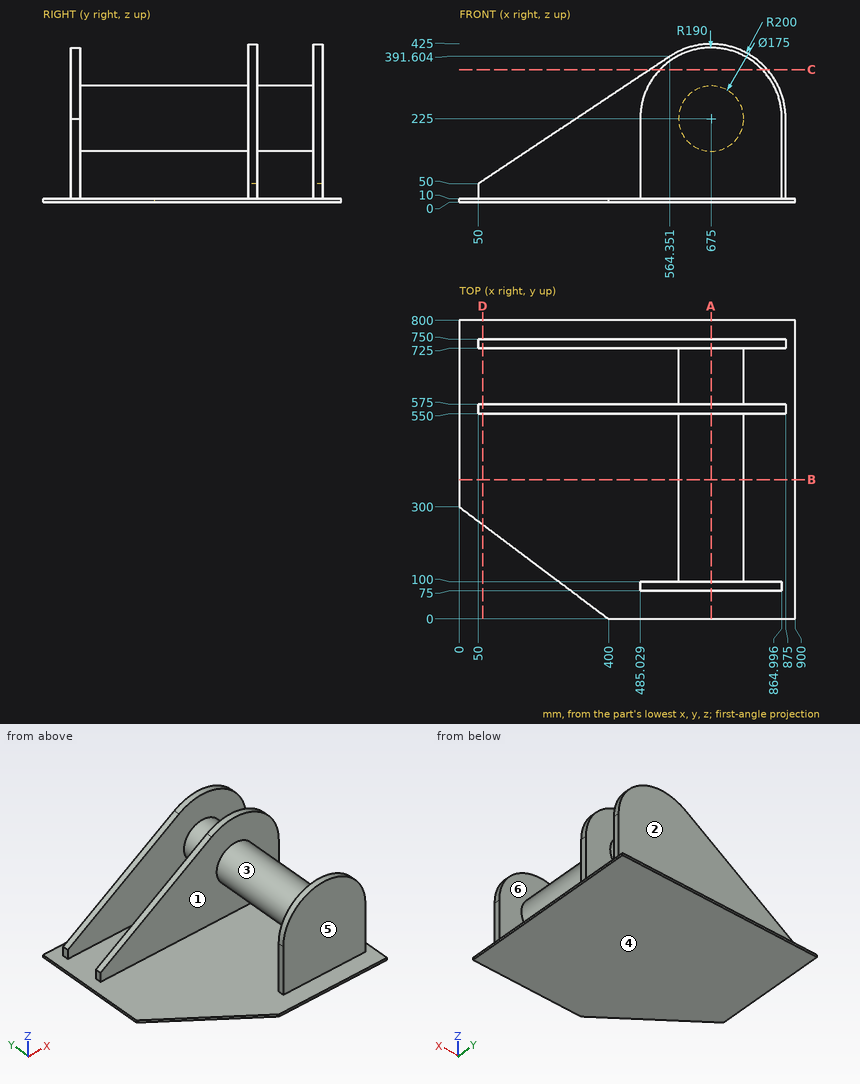
Source: three-view drawing plus pictorial views. Frame: mm from the lowest corner of the part. A direction names the side the tool comes from. Coordinates: 2 decimals unless noted, no trailing zeros. Loops run counter-clockwise (first coordinate to the right, second up) from the corner with the lowest first, then second, coordinate; pieces in that order, holes last. Notation, with made-up numbers: (-8.5, 67) -> (22.5, 67) arc R15 ccw to (22.5, 76) -> close; hole circle Ø3 at (22, 17.5). An arc over 180 degrees is marked (long way). Answer in a Markdown table with one row per item. Add a question column.
Q1. Section C-C on z = 356.5. Return the cut outline in (x, y) (1 decimal).
Q2. Contact query for flat-ended pins moving along their axis: pin 1 Ø7.5 at (y, z) = (739, 168) entering from +X; pin 2 Ø4 at (y, z) = (248.5, 288) entering from +X; pin 3 Ø8 at (x, z) = (613, 293) entering from -Y. Output: stop coordinate, or through.
Q3. Pull-direction query (Z, two-part tool) for the marked faces 1, 2, 3 and 4; classes: pulls with the +Z half, pulls with the -Z half, needs draft (parallel to the pull), parting line crosses it, or undercut.
Q4. Section B-B on y = 373.5. Return the cut outline in (x, z).
Q5. Section D-D on x = 62.5. Return the cut outline in (y, z) (1 decimal).
Q6. Ray query, line 1 along Y through (x, z) = (558, 219.5); line 2 along Y through (x, z) = (211, 128.5); line 3 along Z through (x, y) = (840, 326.5). Return the intervals inside material, ascending.
Q7. Section A-A on x = 675. Return the cut outline in (y, z).
Q8. Reachability of the marked faces 5 and 6 from +Z, -Z, +X, -X, +Y, -Y: full face, straight path, thin tool, end or side. Return the list, or none.
Computed values:
| question | item | result |
|---|---|---|
| 1 | outline | (511.5, 550) -> (825.7, 550) -> (825.7, 575) -> (511.5, 575) -> close; (511.5, 725) -> (825.7, 725) -> (825.7, 750) -> (511.5, 750) -> close; (537.9, 75) -> (812.1, 75) -> (812.1, 100) -> (537.9, 100) -> close |
| 2 | pin 1 | stops at x = 875 |
| 2 | pin 2 | stops at x = 737.73 |
| 2 | pin 3 | stops at y = 75 |
| 3 | face 1 | undercut |
| 3 | face 2 | needs draft |
| 3 | face 3 | undercut |
| 3 | face 4 | pulls with the -Z half |
| 4 | outline | (0, 0) -> (900, 0) -> (900, 10) -> (0, 10) -> close; circle Ø175 at (675, 225) |
| 5 | outline | (253.1, 0) -> (800, 0) -> (800, 10) -> (750, 10) -> (750, 58.3) -> (725, 58.3) -> (725, 10) -> (575, 10) -> (575, 58.3) -> (550, 58.3) -> (550, 10) -> (253.1, 10) -> close |
| 6 | line 1 | y = 75 to 100, 550 to 575, 725 to 750 |
| 6 | line 2 | y = 550 to 575, 725 to 750 |
| 6 | line 3 | z = 0 to 10 |
| 7 | outline | (0, 0) -> (800, 0) -> (800, 10) -> (750, 10) -> (750, 425) -> (725, 425) -> (725, 312.5) -> (575, 312.5) -> (575, 425) -> (550, 425) -> (550, 312.5) -> (100, 312.5) -> (100, 415) -> (75, 415) -> (75, 10) -> (0, 10) -> close; hole (100, 10) -> (550, 10) -> (550, 137.5) -> (100, 137.5) -> close; hole (575, 10) -> (725, 10) -> (725, 137.5) -> (575, 137.5) -> close |
| 8 | face 5 | +Z, +X, -X, -Y |
| 8 | face 6 | none |
